Verification items for the finished model (mm, model axes). A direction names the side the tool comes from. Give positions to 0.01 mm unless a question says otherwise; leave off trailing zeros. Write each loop counter-clockwise with the first axis right and the second up, starting at its lowest first coordinate (ties: lowest second). Pieces come first, ordered by that corner, then holes. Notation, with made-up numbers: (82, 60.5) -> (108, 60.5) arc R9 cw to (108, 75.5) -> close; hole circle Ø8 at (75.5, 9). An arc over 180 degrees is marked (long way). Write item = value, one per line.
from build123d import *

# Parameters (mm, degrees)
F0_R     = 1.25
F1_DEPTH = 10
F3_R     = 3
F3_W     = 16.9056220651
F3_H     = 9.25
F4_DEPTH = 7


with BuildPart() as f1:
    # F0 (on Top) → F1 (new body)
    with BuildSketch(Plane.XY):
        with BuildLine():
            ThreePointArc((32.5, -7.5), (40, 0), (32.5, 7.5))
            Line((32.5, 7.5), (-32.5, 7.5))
            ThreePointArc((-32.5, 7.5), (-40, 0), (-32.5, -7.5))
            Line((-32.5, -7.5), (32.5, -7.5))
        make_face()
        with BuildLine():
            ThreePointArc((-17.4693779349, 1.625), (-15.8443779349, 0), (-17.4693779349, -1.625))
            Line((-17.4693779349, -1.625), (-31.375, -1.625))
            ThreePointArc((-31.375, -1.625), (-33, 0), (-31.375, 1.625))
            Line((-31.375, 1.625), (-17.4693779349, 1.625))
        make_face(mode=Mode.SUBTRACT)
        with Locations((32.5, 0)):
            Circle(F0_R, mode=Mode.SUBTRACT)
    extrude(amount=F1_DEPTH)

    # F3 (on offset) → F4 (cut)
    with BuildSketch(Plane.XY.offset(10)):
        with Locations((32.5, 0)):
            Circle(F3_R)
        with Locations((-24.4221889675, 0)):
            Rectangle(F3_W, F3_H)
        with BuildLine():
            Line((-32.875, -4.625), (-32.875, 4.625))
            ThreePointArc((-32.875, 4.625), (-37.5, 0), (-32.875, -4.625))
        make_face()
        with BuildLine():
            ThreePointArc((-15.9693779349, -4.625), (-11.3443779349, 0), (-15.9693779349, 4.625))
            Line((-15.9693779349, 4.625), (-15.9693779349, -4.625))
        make_face()
    extrude(amount=-F4_DEPTH, mode=Mode.SUBTRACT)


solid = f1.part
Item 1: Mould release check, pull along X, two halves, no side actions. Record for faces 4 (the cylindrical face through (-40, 0, 5)), 5 (the cylindrical face through (-37.5, 0.1, 6.5)), 6 (the flat face through (0, 7.5, 5)), 7 (the cylindrical face through (40, 0, 5)): +X half, -X half, draft (parallel to the pull), parting line (faces both ways), or undercut.
Response values:
face_4 = -X half
face_5 = undercut
face_6 = draft
face_7 = +X half
Item 2: Sectioned sample at B-B on x = -21.5. Record the cut outline in (y, z) (3 decimals), then the cut area to 3 significant figures.
Response values:
outline = (-7.5, 0) -> (-1.625, 0) -> (-1.625, 3) -> (-4.625, 3) -> (-4.625, 10) -> (-7.5, 10) -> close; (1.625, 0) -> (7.5, 0) -> (7.5, 10) -> (4.625, 10) -> (4.625, 3) -> (1.625, 3) -> close
area = 75.5 mm^2
Item 3: Sectioned sample at D-D on z = 1. Record the cut outline in (x, y) (3 decimals), then the cut area to 3 significant figures.
Response values:
outline = (-32.5, -7.5) -> (32.5, -7.5) arc R7.5 ccw to (32.5, 7.5) -> (-32.5, 7.5) arc R7.5 ccw to start; hole (-31.375, -1.625) -> (-17.469, -1.625) arc R1.625 ccw to (-17.469, 1.625) -> (-31.375, 1.625) arc R1.625 ccw to start; hole circle Ø2.5 at (32.5, 0)
area = 1,090 mm^2
Item 4: Sectioned sample at A-A on y = 0. Record the cut outline in (x, z), then the cut area to 3 significant figures.
Response values:
outline = (-40, 0) -> (-33, 0) -> (-33, 3) -> (-37.5, 3) -> (-37.5, 10) -> (-40, 10) -> close; (-15.84, 0) -> (31.25, 0) -> (31.25, 3) -> (29.5, 3) -> (29.5, 10) -> (-11.34, 10) -> (-11.34, 3) -> (-15.84, 3) -> close; (33.75, 0) -> (40, 0) -> (40, 10) -> (35.5, 10) -> (35.5, 3) -> (33.75, 3) -> close
area = 516 mm^2
Item 5: Material ranges on line 1 (X direction, y = 0, z = 0.6); line 2 (Y direction, x = 32.5, z = 0.8); line 3 (Y direction, x = -16.5, z = 4) (3 decimals), recorded low to high.
Response values:
line_1 = -40 to -33, -15.84 to 31.25, 33.75 to 40
line_2 = -7.5 to -1.25, 1.25 to 7.5
line_3 = -7.5 to -4.625, 4.625 to 7.5
Item 6: Go/stop test with flat-tipped pins: P1, Ø4.5, axis at x = -18, y = 2, coming from the +Z side; P2, Ø3, axis at y = 5, z = 2, coming from the -X side. Record where each tip stops, or that it passes through.
Response values:
P1 = 3
P2 = -39.13
Item 7: Sectioned sample at C-C on z = 7. Record the cut outline in (x, y) (3 decimals).
Response values:
outline = (-32.5, -7.5) -> (32.5, -7.5) arc R7.5 ccw to (32.5, 7.5) -> (-32.5, 7.5) arc R7.5 ccw to start; hole (-32.875, -4.625) -> (-15.969, -4.625) arc R4.625 ccw to (-15.969, 4.625) -> (-32.875, 4.625) arc R4.625 ccw to start; hole circle Ø6 at (32.5, 0)
Item 8: Set-up check for faces 1 (the flat face through (-24, -1.625, 1)), 2 (the flat face through (8, 0, 10)), 3 (the cylindrical face through (-11.345, -0.102, 6.549)): record each of +Z, -Z, +X, -X, +Y, -Y from which the full face is reachable in a straight line by a thin tool's end or side.
Response values:
face_1 = +Z, -Z
face_2 = +Z, +X, -X, +Y, -Y
face_3 = +Z
